Design review of the part shown in the three views and the two pictorial views. Dimensions are in mm from the part's minimum x, y and z. Coordinates: 2 decimals unless noted, no trailing zeros. Loops run counter-clockwise (first coordinate to the right, second up) from the corner with the lowest first, then second, coordinate; pieces in that order, holes last. Notation, with made-up numbers: M 84,-32 L 109,-32 A10 cw 109,-27 Z; hole C 73,26 d10. An arc over 180 degrees is marked long. Put each result on its own line as item: value. Start each with the question number.
(1) For probe 1 along Y at (x, z) = (5.5, 12); probe 2 along Y at (x, z) = (2, 16); probe 3 along X at (y, z) = (2.5, 8.5), list the stretches that pass through material, from the lowest coordinate up. Write a range as [from, to].
(2) Clearance check with flat-ended pins moving along their axes: pin 1 (4 mm diameter, centred on y = 9.5, z = 14, fed in from -X); pin 2 (2 mm diameter, centred on y = 10, z = 25.5, fed in from +X). State where each tip first meets the part, or that it passes through.
(3) Take a section at A-A, the plane x = 5.5. Give the boundary of the cut face in (y, z), then the cut area to 3 significant figures.
(4) Take a section at C-C, the plane z = 26.25. Give the boundary of the cut face in (x, y), then the cut area to 3 significant figures.
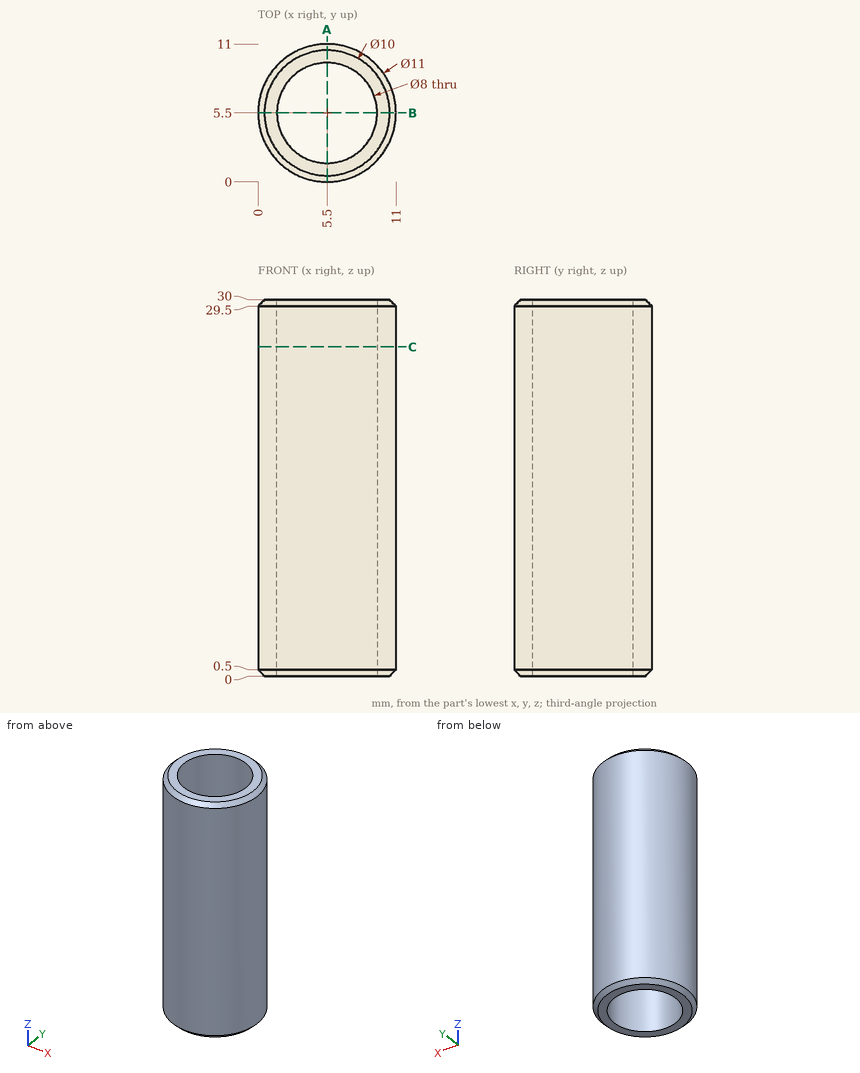
Computed values:
1. probe 1: y = [0, 1.5], [9.5, 11]
1. probe 2: y = [1.26, 3.56], [7.44, 9.74]
1. probe 3: x = [0.89, 2.85], [8.15, 10.11]
2. pin 1: stops at x = 0.38
2. pin 2: stops at x = 9.74
3. outline: M 0,0.5 L 0.5,0 L 1.5,0 L 1.5,30 L 0.5,30 L 0,29.5 Z; M 9.5,0 L 10.5,0 L 11,0.5 L 11,29.5 L 10.5,30 L 9.5,30 Z
3. area: 89.5 mm^2
4. outline: C 5.5,5.5 d11; hole C 5.5,5.5 d8
4. area: 44.8 mm^2
